For this review, take the finished solid that the model builds, in its own axes (mm). Face numbers are marked on the shaded views. Coordinates: 2 decimals unless noted, no trailing zeros. Write each loop counter-clockwise with the first axis right and the second up, starting at its lowest first coordinate (ties: lowest second). Pieces come first, ordered by that corner, then holes.
```python
from build123d import *

# Parameters (mm, degrees)
F0_R     = 3.96875
F1_DEPTH = 3.175
F2_R     = 4.9721039952
F2_W     = 58.7375
F2_H     = 14.2875
F2_H_2   = 3.175
F2_R_2   = 3.96875
F3_DEPTH = 3.175
F4_W     = 3.175
F4_H     = 20.6375
F4_W_2   = 3.96875
F4_H_2   = 14.2875
F4_H_3   = 3.175
F4_W_3   = 47.625
F5_DEPTH = 3.175
F6_DEPTH = 28.575
F7_DEPTH = 1.5875


with BuildPart() as f1:
    # F0 (on Top) → F1 (new body)
    with BuildSketch(Plane.XY):
        with BuildLine():
            Line((12.7, 29.36875), (-12.7, 29.36875))
            Line((-12.7, 29.36875), (-12.7, -29.36875))
            Line((-12.7, -29.36875), (-3.96875, -29.36875))
            Line((-3.96875, -29.36875), (-3.96875, -18.25625))
            ThreePointArc((-3.96875, -18.25625), (0, -14.2875), (3.96875, -18.25625))
            Line((3.96875, -18.25625), (3.96875, -29.36875))
            Line((3.96875, -29.36875), (12.7, -29.36875))
            Line((12.7, -29.36875), (12.7, 29.36875))
        make_face()
        with Locations((0, 16.66875)):
            Circle(F0_R, mode=Mode.SUBTRACT)
    extrude(amount=F1_DEPTH)

    # F2 (on face) → F3 (join)
    with BuildSketch(Plane(origin=(-12.7, 0, 0), x_dir=(0, -1, 0), z_dir=(-1, 0, 0))):
        with BuildLine():
            Line((-29.36875, 38.1), (-29.36875, 17.4625))
            Line((-29.36875, 17.4625), (29.36875, 17.4625))
            Line((29.36875, 17.4625), (-22.0211824404, 45.2408418597))
            ThreePointArc((-22.0211824404, 45.2408418597), (-27.2038122264, 43.2229476746), (-29.36875, 38.1))
        make_face()
        with Locations((-22.225, 38.1)):
            Circle(F2_R, mode=Mode.SUBTRACT)
        with Locations((0, 10.31875)):
            Rectangle(F2_W, F2_H)
        with Locations((0, 1.5875)):
            Rectangle(F2_W, F2_H_2)
        with Locations((-22.225, 38.1)):
            Circle(F2_R)
        with Locations((-22.225, 38.1)):
            Circle(F2_R_2, mode=Mode.SUBTRACT)
    extrude(amount=-F3_DEPTH)

    # F4 (on face) → F5 (join)
    with BuildSketch(Plane.YZ.offset(12.7)):
        Polygon((-29.36875, 17.4625), (18.25625, 17.4625), (18.25625, 38.1), (8.810625, 38.1), align=None)
        Polygon((8.810625, 38.1), (18.25625, 38.1), (18.25625, 43.2057432432), align=None)
        with BuildLine():
            ThreePointArc((18.25625, 38.1), (19.4186699622, 40.9063300378), (22.225, 42.06875))
            Line((22.225, 42.06875), (22.225, 45.24375))
            ThreePointArc((22.225, 45.24375), (22.1230808471, 45.2430229279), (22.0211824404, 45.2408418597))
            Line((22.0211824404, 45.2408418597), (18.25625, 43.2057432432))
            Line((18.25625, 43.2057432432), (18.25625, 38.1))
        make_face()
        with BuildLine():
            ThreePointArc((22.225, 42.06875), (25.0313300378, 40.9063300378), (26.19375, 38.1))
            Line((26.19375, 38.1), (26.19375, 44.0398811015))
            ThreePointArc((26.19375, 44.0398811015), (24.2986608261, 44.9361608261), (22.225, 45.24375))
            Line((22.225, 45.24375), (22.225, 42.06875))
        make_face()
        with BuildLine():
            Line((26.19375, 38.1), (29.36875, 38.1))
            ThreePointArc((29.36875, 38.1), (28.5251953095, 41.4675960454), (26.19375, 44.0398811015))
            Line((26.19375, 44.0398811015), (26.19375, 38.1))
        make_face()
        with Locations((27.78125, 27.78125)):
            Rectangle(F4_W, F4_H)
        with BuildLine():
            Line((22.225, 17.4625), (26.19375, 17.4625))
            Line((26.19375, 17.4625), (26.19375, 38.1))
            ThreePointArc((26.19375, 38.1), (25.0313300378, 35.2936699622), (22.225, 34.13125))
            Line((22.225, 34.13125), (22.225, 17.4625))
        make_face()
        with BuildLine():
            Line((18.25625, 17.4625), (22.225, 17.4625))
            Line((22.225, 17.4625), (22.225, 34.13125))
            ThreePointArc((22.225, 34.13125), (19.4186699622, 35.2936699622), (18.25625, 38.1))
            Line((18.25625, 38.1), (18.25625, 17.4625))
        make_face()
        with Locations((20.240625, 10.31875)):
            Rectangle(F4_W_2, F4_H_2)
        with Locations((24.209375, 10.31875)):
            Rectangle(F4_W_2, F4_H_2)
        with Locations((27.78125, 10.31875)):
            Rectangle(F4_W, F4_H_2)
        with Locations((27.78125, 1.5875)):
            Rectangle(F4_W, F4_H_3)
        with Locations((24.209375, 1.5875)):
            Rectangle(F4_W_2, F4_H_3)
        with Locations((20.240625, 1.5875)):
            Rectangle(F4_W_2, F4_H_3)
        with Locations((-5.55625, 1.5875)):
            Rectangle(F4_W_3, F4_H_3)
        with Locations((-5.55625, 10.31875)):
            Rectangle(F4_W_3, F4_H_2)
    extrude(amount=-F5_DEPTH)

    # F2 (on face) → F6 (join)
    with BuildSketch(Plane(origin=(-12.7, 0, 0), x_dir=(0, -1, 0), z_dir=(-1, 0, 0))):
        with Locations((-22.225, 38.1)):
            Circle(F2_R_2)
    extrude(amount=-F6_DEPTH)

    # F2 (on face) → F7 (join)
    with BuildSketch(Plane(origin=(-12.7, 0, 0), x_dir=(0, -1, 0), z_dir=(-1, 0, 0))):
        with Locations((-22.225, 38.1)):
            Circle(F2_R)
        with Locations((-22.225, 38.1)):
            Circle(F2_R_2, mode=Mode.SUBTRACT)
        with Locations((-22.225, 38.1)):
            Circle(F2_R_2)
    extrude(amount=F7_DEPTH)


solid = f1.part
```
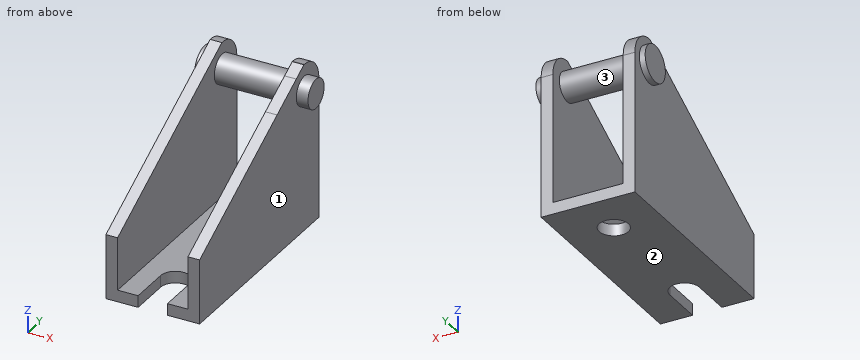
Q1. Add section C-C (x = 12). State the section outline as (y, z) points (1 decimal).
Ans:
outline: (-29.4, 0) - (29.4, 0) - (29.4, 38.1) arc R7.1 ccw to (22, 45.2) - (-29.4, 17.5) - close
Q2. For probe 1 along X at (y, z) = (-2.5, 18) (3 decimals); probe 2 along Y at (x, z) = (0, 2.2); probe 3 along Z at (x, y) = (-9, 21.5) (3 decimals), list the stretches that pass through material, from the lowest coordinate up.
Ans:
probe 1: x = -12.7 to -9.525, 9.525 to 12.7
probe 2: y = -14.29 to 12.7, 20.64 to 29.37
probe 3: z = 0 to 3.175, 34.198 to 42.002
Q3. Add section B-B (z = 15). State the section outline as (x, y) points (3 decimals).
Ans:
outline: (-12.7, -29.369) - (-9.525, -29.369) - (-9.525, 29.369) - (-12.7, 29.369) - close; (9.525, -29.369) - (12.7, -29.369) - (12.7, 29.369) - (9.525, 29.369) - close
Q4. Draft analysis for pull direction Z (two halves, no side actions). For the marked faces 1, 2 and 3, state which applies: +Z half, -Z half, draft (parallel to the pull), parting line (faces both ways), or undercut.
Ans:
face 1: draft
face 2: -Z half
face 3: undercut
Q5. Clearance check with flat-ended pins moving along their axes: pin 1 Ø10 at (x, z) = (-8, 8) entering from -Y; pin 2 Ø12 at (y, z) = (-0.5, 6) entering from -X; pin 3 Ø5.5 at (x, y) = (-3, -3.5) entering from +Z (3 decimals); pin 4 Ø12.5 at (y, z) = (5.5, 26) entering from +X. State where each tip first meets the part, or that it passes through.
Ans:
pin 1: stops at y = -29.37
pin 2: stops at x = -12.7
pin 3: stops at z = 3.175
pin 4: stops at x = 12.7
Q6. Add section A-A (x = 0). State the section outline as (y, z) points (1 decimal).
Ans:
outline: (-14.3, 0) - (12.7, 0) - (12.7, 3.2) - (-14.3, 3.2) - close; circle Ø7.9 at (22.2, 38.1); (20.6, 0) - (29.4, 0) - (29.4, 3.2) - (20.6, 3.2) - close
